The model under review builds one solid part; all positions refer to its coordinate system, in mm. A direction names the side the tool comes from. Round coordinates to 2 decimals unless told otherwise and drop trailing zeros. Order: outer loops, then holes, each group sorted by start corner. A loop starts at its lowest first (then second) coordinate and runs counter-clockwise, first axis right, second up. Notation, with made-up numbers: M 5,9.25 L 32,9.25 A20 cw 32,27.25 Z; hole C 70,-15 d1. An arc over 180 degrees is marked long. Answer as a JSON object with one key per item and string values. Group by question number.
1) Consider section A-A, the plane x = -21.25. Write out the cut boundary in (y, z).
2) To check wall thickness, follow line 1 (X direction, y = -7.6, z = 0); line 2 (Z direction, x = 21.25, y = -8.25); line 3 (X direction, y = -6.5, z = 2). State the ranges of each line that lie inside material, in increasing order.
3) Consider section C-C, the plane z = -3.75. Write out the cut boundary in (x, y), then the cut area to 3 significant figures.
4) For faces 1 (the flat face through (13.75, -5, 0)), 2 (the flat face through (-26.25, -8, 0)), 3 (the flat face through (-21, -9.1, 0)), list the 3-axis set-ups (+Z, -Z, +X, -X, +Y, -Y) from which the entire face can be reached by the end or side of a thin tool; tool diameter is ignored.
5) Consider section D-D, the plane x = -1. Write out the cut boundary in (y, z).
6) The part is to be moulded in two halves that separate along Z. For faces 4 (the cylindrical face through (24.067, -7.655, 1.168)), 5 (the cylindrical face through (-25.65, -7.97, 4.43)), 6 (the cylindrical face through (-18.433, -7.655, 1.168)), 7 (the flat face through (17.8, -6, 0.1)), say which applies: +Z half, -Z half, draft (parallel to the pull), parting line (faces both ways), or undercut.
7) Insertion check: pin 1 Ø6 at (x, z) = (-17.5, 3.5) entering from +Y; pin 2 Ø1.1 at (y, z) = (-4, 1.5) entering from +X; pin 3 Ø3 at (x, z) = (22, 0.5) entering from +Y. Each pin has a flat end and moves straight along its axis. Give the tip position at first contact, or say it passes through.
```python
from build123d import *

# Parameters (mm, degrees)
BOSS_EXTRUDE1_DEPTH = 5
FILLET1_R           = 2
FILLET2_R           = 5
FILLET3_R           = 2
FILLET4_R           = 2
SKETCH3_R           = 3.05
CUT_EXTRUDE1_DEPTH  = 3.1
CHAMFER1_SIZE       = 0.25


with BuildPart() as part:
    # Sketch1 → Boss-Extrude1 (new body, symmetric)
    with BuildSketch(Plane.XY):
        Polygon((-16.25, 2.5), (16.25, 2.5), (16.25, -6), (26.25, -6), (26.25, -10), (16.25, -10), (13.75, -10), (13.75, 0), (-13.75, 0), (-13.75, -10), (-16.25, -10), (-26.25, -10), (-26.25, -6), (-16.25, -6), align=None)
    extrude(amount=BOSS_EXTRUDE1_DEPTH, both=True)

    # Fillet1
    fillet1_edges = [part.edges().sort_by_distance(p)[0] for p in [
        (13.75, 0, 0),
        (-13.75, 0, 0),
    ]]
    fillet(fillet1_edges, radius=FILLET1_R)

    # Fillet2
    fillet2_edges = [part.edges().sort_by_distance(p)[0] for p in [
        (-16.25, 2.5, 0),
        (16.25, 2.5, 0),
    ]]
    fillet(fillet2_edges, radius=FILLET2_R)

    # Fillet3
    fillet3_edges = [part.edges().sort_by_distance(p)[0] for p in [
        (26.25, -8, -5),
        (-26.25, -8, -5),
        (-26.25, -8, 5),
        (26.25, -8, 5),
    ]]
    fillet(fillet3_edges, radius=FILLET3_R)

    # Fillet4
    fillet4_edges = [part.edges().sort_by_distance(p)[0] for p in [
        (13.75, -10, 0),
        (-13.75, -10, 0),
    ]]
    fillet(fillet4_edges, radius=FILLET4_R)

    # Sketch3 → Cut-Extrude1 (cut)
    with BuildSketch(Plane(origin=(0, -6, 0), x_dir=(1, 0, 0), z_dir=(0, 1, 0))):
        with Locations((21.25, 0)):
            Circle(SKETCH3_R)
        with Locations((-21.25, 0)):
            Circle(SKETCH3_R)
    extrude(amount=-CUT_EXTRUDE1_DEPTH, mode=Mode.SUBTRACT)

    # Chamfer1
    chamfer1_edges = [part.edges().sort_by_distance(p)[0] for p in [
        (18.2, -6, 0),
        (-24.3, -6, 0),
    ]]
    chamfer(chamfer1_edges, length=CHAMFER1_SIZE)


solid = part.part
```
Results list:
{
 "1": {"outline": "M -10,-5 L -6,-5 L -6,-3.3 L -6.25,-3.05 L -9.1,-3.05 L -9.1,3.05 L -6.25,3.05 L -6,3.3 L -6,5 L -10,5 Z"},
 "2": {"line 1": "-26.25 to -24.3, -18.2 to -13.75, 13.75 to 18.2, 24.3 to 26.25", "line 2": "-5 to -3.05, 3.05 to 5", "line 3": "-26.25 to -23.55, -18.95 to -13.75, 13.75 to 18.95, 23.55 to 26.25"},
 "3": {"outline": "M -26.1,-10 L -15.75,-10 A2 ccw -13.75,-8 L -13.75,-2 A2 cw -11.75,0 L 11.75,0 A2 cw 13.75,-2 L 13.75,-8 A2 ccw 15.75,-10 L 26.1,-10 L 26.1,-6 L 16.25,-6 L 16.25,-2.5 A5 ccw 11.25,2.5 L -11.25,2.5 A5 ccw -16.25,-2.5 L -16.25,-6 L -26.1,-6 Z", "area": "199 mm^2"},
 "4": {"face 1": "+Z, -Z, -Y", "face 2": "+Z, -Z, -X, +Y, -Y", "face 3": "+Y"},
 "5": {"outline": "M 0,-5 L 2.5,-5 L 2.5,5 L 0,5 Z"},
 "6": {"face 4": "undercut", "face 5": "+Z half", "face 6": "undercut", "face 7": "draft"},
 "7": {"pin 1": "y = 1.3", "pin 2": "x = 16.25", "pin 3": "y = -9.1"}
}
